Model file for the job. Use its own axes, mm. A direction names the side the tool comes from. Round coordinates to 2 decimals unless told otherwise and drop trailing zeros. Order: outer loops, then holes, each group sorted by start corner. A loop starts at its lowest first (then second) coordinate and runs counter-clockwise, first axis right, second up. Notation, with made-up numbers: (73.5, 44) -> (95.5, 44) arc R15 ccw to (95.5, 58) -> close; hole circle Ø2 at (84.25, 60). An arc over 180 degrees is marked (long way). Put each result on its own line as item: value. Start each with the question number.
Q1. Pull direction X, two halves, no side cores. Call faces 4 (the face through (49, 20, 43)), 5 (the face through (0.9, 21.7, 4.1)), 6 (the face through (-69.15, 4.93, -21.78)): released by +X, released by -X, zero draft, split by the parting line, or undercut.
Q2. Probe L1, parallel to X at y = 4.5, z = 0; L2, parallel to Z at x = -22.5, y = 12.75; L3, parallel to Z at x = 3, y = 22. List the from-to ranges inside material, lowest first.
Q3. Flat gauge pins, fed straight in: P1, Ø5.5, axis at x = -0.5, z = 0.5, coming from the +Y side; P2, Ø4, axis at x = 22.5, z = -38.97, coming from the -Y side; P3, Ø1, axis at y = 41.5, z = -6.5, coming from the +X side; P4, Ø5, axis at x = -6, y = 41.5, coming from the -Z side. Where does each tip first touch, or does it go through?
Q4. Cut at B-B, the plane x = -45. List the corners of the cut face in (y, z).
Q5. Cut at D-D, the plane z = 51. List the corners of the cut face in (x, y).
Q6. Cut at A-A, the plane y = 26. List the corners of the cut face in (x, z).
Q7. 3-axis set-ups, long thin cutter, end or side, ignore diameter. For faces 1 (the face through (-61.522, 14.93, -19.374)), 2 (the face through (-69.15, 44.93, -21.78)), 3 (the face through (37, 20, 22)): which of +Z, -Z, +X, -X, +Y, -Y reach the whole face in a straight line?
from build123d import *

# Parameters (mm, degrees)
SKETCH2_R          = 2.5
CUT_EXTRUDE1_DEPTH = 30


with BuildPart() as part:
    # Sketch1 → Revolve1 (revolve)
    with BuildSketch(Plane.XY):
        Polygon((-72.5, 0), (0, 0), (0, 20), (-2.5, 20), (-12.5, 30), (-22.5, 20), (-32.5, 30), (-42.5, 20), (-47.5, 20), (-47.5, 50), (-72.5, 50), (-72.5, 40), (-65.326285386, 40), (-65.326285386, 30), (-72.5, 30), (-72.5, 20), (-64.5, 20), (-64.5, 10), (-72.5, 10), align=None)
    revolve(axis=Axis((0, 20, 0), (0, -1, 0)))

    # Sketch2 → Cut-Extrude1 (cut)
    with BuildSketch(Plane.XZ):
        with BuildLine():
            ThreePointArc((-47.5, 0), (-45, -2.5), (-42.5, 0))
            Line((-42.5, 0), (-47.5, 0))
        make_face()
        with BuildLine():
            Line((-47.5, 0), (-42.5, 0))
            ThreePointArc((-42.5, 0), (-45, 2.5), (-47.5, 0))
        make_face()
        with Locations((-22.5, -38.97114317)):
            Circle(SKETCH2_R)
        with Locations((-22.5, 38.97114317)):
            Circle(SKETCH2_R)
        with Locations((22.5, 38.97114317)):
            Circle(SKETCH2_R)
        with Locations((45, 0)):
            Circle(SKETCH2_R)
        with Locations((22.5, -38.97114317)):
            Circle(SKETCH2_R)
    extrude(amount=-CUT_EXTRUDE1_DEPTH, mode=Mode.SUBTRACT)


solid = part.part
Ans:
1. face 4: zero draft
1. face 5: undercut
1. face 6: split by the parting line
2. L1: x = -72.5 to -47.5, -42.5 to 42.5, 47.5 to 72.5
2. L2: z = -60.45 to -41.47, -36.47 to 36.47, 41.47 to 60.45
2. L3: z = -72.44 to -47.41, -40.39 to -24.32, -20.28 to -3.35, 3.35 to 20.28, 24.32 to 40.39, 47.41 to 72.44
3. P1: stops at y = 20.96
3. P2: passes through
3. P3: stops at x = 72.25
3. P4: stops at z = -72.42
4. outline: (0, -56.84) -> (10, -56.84) -> (10, -46.21) -> (20, -46.21) -> (20, -56.84) -> (30, -56.84) -> (30, -47.36) -> (40, -47.36) -> (40, -56.84) -> (50, -56.84) -> (50, -15.21) -> (20, -15.21) -> (20, -2.5) -> (0, -2.5) -> close; (0, 2.5) -> (20, 2.5) -> (20, 15.21) -> (50, 15.21) -> (50, 56.84) -> (40, 56.84) -> (40, 47.36) -> (30, 47.36) -> (30, 56.84) -> (20, 56.84) -> (20, 46.21) -> (10, 46.21) -> (10, 56.84) -> (0, 56.84) -> close
5. outline: (-51.53, 0) -> (51.53, 0) -> (51.53, 10) -> (39.49, 10) -> (39.49, 20) -> (51.53, 20) -> (51.53, 30) -> (40.82, 30) -> (40.82, 40) -> (51.53, 40) -> (51.53, 50) -> (-51.53, 50) -> (-51.53, 40) -> (-40.82, 40) -> (-40.82, 30) -> (-51.53, 30) -> (-51.53, 20) -> (-39.49, 20) -> (-39.49, 10) -> (-51.53, 10) -> close
6. outline: circle Ø145 at (0, 0); circle Ø73 at (0, 0); circle Ø33 at (0, 0); hole circle Ø95 at (0, 0); hole circle Ø57 at (0, 0); hole circle Ø17 at (0, 0)
7. face 1: none
7. face 2: +Y, -Y
7. face 3: +Y
